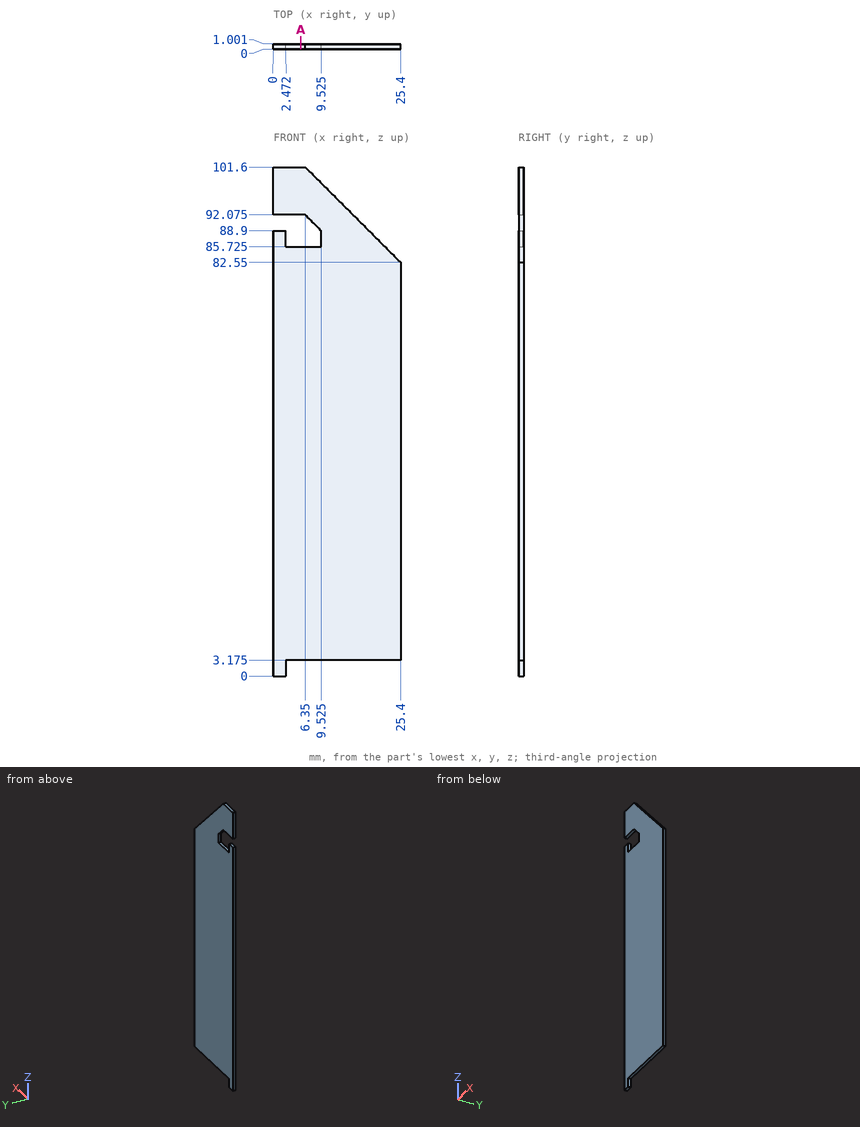
Design review of the part shown in the three views and the two pictorial views. Dimensions are in mm from the part's minimum x, y and z. Coordinates: 2 decimals unless noted, no trailing zeros. Order: outer loops, then holes, each group sorted by start corner. A loop starts at its lowest first (then second) coordinate and runs counter-clockwise, first axis right, second up.
1) Wall thickness on line 1 along Z through (x, y) = (9.25, 0.5) (1 decimal); line 2 along Z through (x, y) = (17.25, 0.65) (1 decimal); line 3 along Z through (x, y) = (22.75, 0.5) (1 decimal): over which ranges is each line inside the solid? List them lowest first.
2) Take a section at A-A, the plane x = 5.5. Give the boundary of the cut face in (y, z) (1 decimal).
3) Clearance check with a flat-ended pin moving along its axis: pin 1 (0.5 mm diameter, centred on y = 0.5, z = 2, fed in from +X). State where the tip first meets the part, or that it passes through.
Returned:
1. line 1: z = 3.2 to 85.7, 89.2 to 98.7
1. line 2: z = 3.2 to 90.7
1. line 3: z = 3.2 to 85.2
2. outline: (0, 3.2) - (1, 3.2) - (1, 85.7) - (0, 85.7) - close; (0, 92.1) - (1, 92.1) - (1, 101.6) - (0, 101.6) - close
3. pin 1: stops at x = 2.47
